For this review, take the finished solid that the model builds, in its own axes (mm). A direction names the side the tool comes from. Give positions to 0.01 mm unless a question says otherwise; leave off trailing zeros. Write each loop counter-clockwise with the first axis right and the second up, starting at its lowest first coordinate (ties: lowest second). Pieces come first, ordered by that corner, then holes. Notation, with made-up numbers: M 33,-36.75 L 74,-36.75 A13 cw 74,-22.75 Z; hole C 81,-29.75 d2. An arc over 180 degrees is marked long. Write item = value, one per line.
Autodesk Inventor part; units mm, degrees
ref_plane "YZ Plane" through (0, 0, 0) normal (1, 0, 0) x (0, 1, 0)
ref_plane "XZ Plane" through (0, 0, 0) normal (0, 1, 0) x (-1, 0, 0)
ref_plane "XY Plane" through (0, 0, 0) normal (0, 0, 1) x (1, 0, 0)
sketch "Sketch1" plane through (0, 0, 0) normal (0, 1, 0) x (-1, 0, 0)
  circle A0 centre (0, 0) radius 2.25
  dimension "d0" = 4.5
extrude "Extrusion1" add sketch "Sketch1" along normal blind 2.5
sketch "Sketch2" plane through (0, 2.5, 0) normal (0, 1, 0) x (1, 0, 0)
  circle A0 centre (0, 0) radius 1
  dimension "d3" = 2
extrude "Extrusion2" add sketch "Sketch2" along normal blind 5
sketch "Sketch3" plane through (0, 0, 0) normal (0, -1, 0) x (1, 0, 0)
  line L0 (0, -1.1547) -> (-1, -0.5774)
  line L1 (-1, -0.5774) -> (-1, 0.5774)
  line L2 (-1, 0.5774) -> (0, 1.1547)
  line L3 (0, 1.1547) -> (1, 0.5774)
  line L4 (1, 0.5774) -> (1, -0.5774)
  line L5 (1, -0.5774) -> (0, -1.1547)
  point P0 (0, 0)
  point P1 (0, 0)
  dimension "d6" = 2
extrude "Extrusion3" cut sketch "Sketch3" against normal blind 1
properties part number "m2_bolt_5mm" material "Stainless Steel"
1. We need section D-D, the plane x = 1.85. Write out the cut boundary in (y, z).
Responses:
outline = M 0,-1.28 L 2.5,-1.28 L 2.5,1.28 L 0,1.28 Z
2. We need section B-B, the plane y = 2.75. Write out the cut boundary in (x, z).
Responses:
outline = C 0,0 d2
3. We need section C-C, the plane z = 0. Write out the cut boundary in (x, y).
Responses:
outline = M -2.25,0 L -1,0 L -1,1 L 1,1 L 1,0 L 2.25,0 L 2.25,2.5 L 1,2.5 L 1,7.5 L -1,7.5 L -1,2.5 L -2.25,2.5 Z
4. We need section A-A, the plane z = 0.8. Write out the cut boundary in (x, y).
Responses:
outline = M -2.1,0 L -0.61,0 L -0.61,1 L 0.61,1 L 0.61,0 L 2.1,0 L 2.1,2.5 L 0.6,2.5 L 0.6,7.5 L -0.6,7.5 L -0.6,2.5 L -2.1,2.5 Z
5. The part is to be moulded in two halves that separate along X. For faces 1 (the face through (0.51, 0.49, -0.86)), 2 (the face through (1, 2.5, -1)), 3 (the face through (0.29, 1.23, -2.23)), say which applies: +X half, -X half, draft (parallel to the pull), parting line (faces both ways), or undercut.
Responses:
face_1 = undercut
face_2 = draft
face_3 = parting line
6. Machinability: for faces 4 (the face through (1, 0, -1)), 5 (the face through (-1, 0.5, 0)), 6 (the face through (0, 5, -1)), which of the approach directions +Z, -Z, +X, -X, +Y, -Y give a long, thin tool a straight path to every point of the face, cutting with its end or side? Answer none if there is none.
Responses:
face_4 = +Z, -Z, +X, -X, -Y
face_5 = -Y
face_6 = +Y
7. Insertion check: P1, Ø1, axis at y = 6, z = -1, coming from the -X side; P2, Ø1.5, axis at y = 5.5, z = -1.5, coming from the -X side; P3, Ø2, axis at y = 5, z = 1, coming from the -X side. Each pin has a flat end and moves straight along its axis. Give the tip position at first contact, or say it passes through.
Responses:
P1 = -0.87
P2 = -0.66
P3 = -1
8. For line 1 along Y through (x, z) = (-1.45, -1.15); line 2 along X through (y, z) = (0.5, 0.3); line 3 along Z through (x, y) = (-0.55, 0.75), list the stretches that pass through material, from the lowest coordinate up. Write a range as from..to.
Responses:
line_1 = 0..2.5
line_2 = -2.23..-1, 1..2.23
line_3 = -2.18..-0.84, 0.84..2.18
